```python
from build123d import *

# Parameters (mm, degrees)
F1_DEPTH = 76.2
F2_R     = 6.35
F3_R     = 12.7


with BuildPart() as f1:
    # F0 (on Right) → F1 (new body, symmetric)
    with BuildSketch(Plane.YZ):
        Polygon((-6.35, 88.9), (-6.35, -6.35), (31.75, -6.35), (31.75, 0), (0, 0), (0, 88.9), align=None)
    extrude(amount=F1_DEPTH, both=True)

    # F2
    f2_edges = [f1.edges().sort_by_distance(p)[0] for p in [
        (0, 0, 0),
    ]]
    fillet(f2_edges, radius=F2_R)

    # F3
    f3_edges = [f1.edges().sort_by_distance(p)[0] for p in [
        (0, -6.35, -6.35),
    ]]
    fillet(f3_edges, radius=F3_R)


solid = f1.part
```
Here's how the part is built. I have some questions about the finished solid (model axes, mm). A direction names the side the tool comes from. Round coordinates to 2 decimals unless told otherwise and drop trailing zeros. Order: outer loops, then holes, each group sorted by start corner. A loop starts at its lowest first (then second) coordinate and runs counter-clockwise, first axis right, second up. Notation, with made-up numbers: (-5.5, 62.25) -> (26.5, 62.25) arc R22 cw to (26.5, 72.25) -> close; hole circle Ø4 at (62.5, -36.5). An arc over 180 degrees is marked (long way). Use a Markdown table: item, result. Add a question column.
(1) I need wall thicknesses on line 1 along Z through (x, y) = (38.5, 13); line 2 along Z through (x, y) = (41, 5.5). Which ranges of each line are inside material? Lowest first, please.
(2) Suppose I cut it at B-B, the plane z = 25. Please give me the cut outline in (x, y), and give its area (3 significant figures).
(3) Suppose I cut it at A-A, the plane x = 61. Please give me the cut outline in (y, z), and give its area (3 significant figures).
(4) For pin 1 Ø4 at (x, y) = (-48, 1.5) entering from -Z; pin 2 Ø5 at (x, y) = (-30, 13.5) entering from +Z; pin 3 Ø3 at (x, z) = (-44, 74) entering from +Y, each with a flat end and sliding along its axis, tell me the tip position at first contact or that it passes through.
(5) For faces 1 (the face through (1, 31.75, -3)), 2 (the face through (1, 19, 0)), which set-ups out of +Z, -Z, +X, -X, +Y, -Y let a thin tool reach every point of the face, with its end or its side?
Verdict:
| question | item | result |
|---|---|---|
| 1 | line 1 | -6.35 to 0 |
| 1 | line 2 | -6.32 to 0.06 |
| 2 | outline | (-76.2, -6.35) -> (76.2, -6.35) -> (76.2, 0) -> (-76.2, 0) -> close |
| 2 | area | 968 mm2 |
| 3 | outline | (-6.35, 6.35) arc R12.7 ccw to (6.35, -6.35) -> (31.75, -6.35) -> (31.75, 0) -> (6.35, 0) arc R6.35 cw to (0, 6.35) -> (0, 88.9) -> (-6.35, 88.9) -> close |
| 3 | area | 780 mm2 |
| 4 | pin 1 | z = -6.03 |
| 4 | pin 2 | z = 0 |
| 4 | pin 3 | y = 0 |
| 5 | face 1 | +Z, -Z, +X, -X, +Y |
| 5 | face 2 | +Z, +X, -X, +Y |
